from build123d import *

# Parameters (mm, degrees)
SKETCH1_R             = 22
SKETCH1_R_2           = 4
BOSS_EXTRUDE1_DEPTH   = 35
BOSS_EXTRUDE2_START   = 10
BOSS_EXTRUDE2_DEPTH   = 15
BOSS_EXTRUDE2_2_DEPTH = 15
BOSS_EXTRUDE2_3_DEPTH = 15
BOSS_EXTRUDE2_4_DEPTH = 15
SKETCH1_4_R           = 30
SKETCH1_4_R_2         = 15
SKETCH1_4_R_3         = 25
SKETCH1_4_R_4         = 10.5
BOSS_EXTRUDE3_DEPTH   = 35
BOSS_EXTRUDE5_START   = 11
BOSS_EXTRUDE5_DEPTH   = 11
SKETCH1_7_R           = 50
SKETCH1_7_R_2         = 22
BOSS_EXTRUDE6_DEPTH   = 35


with BuildPart() as part:
    # Sketch1 → Boss-Extrude1 (new body)
    with BuildSketch(Plane(origin=(0, 0, 0), x_dir=(1, 0, 0), z_dir=(0, 1, 0))):
        with Locations(Location((0, 0, 0), (0, 0, 270))):
            Circle(SKETCH1_R)
        with Locations(Location((-11.727472237, 9.352347028, 0), (0, 0, 270))):
            Circle(SKETCH1_R_2, mode=Mode.SUBTRACT)
        with Locations(Location((-14.623918683, -3.337814009, 0), (0, 0, 270))):
            Circle(SKETCH1_R_2, mode=Mode.SUBTRACT)
        with Locations(Location((-6.508256087, -13.514533019, 0), (0, 0, 270))):
            Circle(SKETCH1_R_2, mode=Mode.SUBTRACT)
        with Locations(Location((6.508256087, -13.514533019, 0), (0, 0, 270))):
            Circle(SKETCH1_R_2, mode=Mode.SUBTRACT)
        with Locations(Location((14.623918683, -3.337814009, 0), (0, 0, 270))):
            Circle(SKETCH1_R_2, mode=Mode.SUBTRACT)
        with Locations(Location((11.727472237, 9.352347028, 0), (0, 0, 270))):
            Circle(SKETCH1_R_2, mode=Mode.SUBTRACT)
        with Locations(Location((0, 15, 0), (0, 0, 270))):
            Circle(SKETCH1_R_2, mode=Mode.SUBTRACT)
    extrude(amount=BOSS_EXTRUDE1_DEPTH)



with BuildPart() as body_2:
    # Sketch1_3 → Boss-Extrude2 (new body)
    with BuildSketch(Plane(origin=(0, 0, 0), x_dir=(1, 0, 0), z_dir=(0, 1, 0)).offset(BOSS_EXTRUDE2_START)):
        with BuildLine():
            Line((-29.090909091, 49.166608302), (-135.454545455, 29.499964981))
            ThreePointArc((-135.454545455, 29.499964981), (-118.841537744, 27.847598103), (-105.684210842, 17.57106706))
            ThreePointArc((-105.684210842, 17.57106706), (-106.272845666, 22.359321946), (-102.540670225, 25.416239066))
            Line((-102.540670225, 25.416239066), (-68.238836594, 31.758650348))
            ThreePointArc((-68.238836594, 31.758650348), (-64.040683205, 30.607898174), (-62.335471097, 26.602779686))
            ThreePointArc((-62.335471097, 26.602779686), (-48.07934713, 41.370886681), (-29.090909091, 49.166608302))
        make_face()
    extrude(amount=BOSS_EXTRUDE2_DEPTH)



with BuildPart() as body_3:
    # Sketch1_3 → Boss-Extrude2 2 (new body)
    with BuildSketch(Plane(origin=(0, 0, 0), x_dir=(1, 0, 0), z_dir=(0, 1, 0)).offset(BOSS_EXTRUDE2_START)):
        with BuildLine():
            Line((65.058027183, 118.797588822), (-29.090909091, 49.166608302))
            ThreePointArc((-29.090909091, 49.166608302), (-14.295406408, 49.673510163), (0, 45.82575695))
            ThreePointArc((0, 45.82575695), (-2.026867504, 49.845767293), (0, 53.865777636))
            Line((0, 53.865777636), (50.073723573, 90.899467114))
            ThreePointArc((50.073723573, 90.899467114), (53.176128361, 91.877785359), (56.223814659, 90.740406669))
            ThreePointArc((56.223814659, 90.740406669), (56.077798236, 106.205763396), (65.058027183, 118.797588822))
        make_face()
    extrude(amount=BOSS_EXTRUDE2_2_DEPTH)


with BuildPart() as body_4:
    # Sketch1_3 → Boss-Extrude2 3 (new body)
    with BuildSketch(Plane(origin=(0, 0, 0), x_dir=(1, 0, 0), z_dir=(0, 1, 0)).offset(BOSS_EXTRUDE2_START)):
        with BuildLine():
            ThreePointArc((-105.684210842, -17.57106706), (-118.841537744, -27.847598103), (-135.454545455, -29.499964981))
            Line((-135.454545455, -29.499964981), (-29.090909091, -49.166608302))
            ThreePointArc((-29.090909091, -49.166608302), (-48.07934713, -41.370886681), (-62.335471097, -26.602779686))
            ThreePointArc((-62.335471097, -26.602779686), (-64.040683205, -30.607898174), (-68.238836594, -31.758650348))
            Line((-68.238836594, -31.758650348), (-102.540670225, -25.416239066))
            ThreePointArc((-102.540670225, -25.416239066), (-106.272845666, -22.359321946), (-105.684210842, -17.57106706))
        make_face()
    extrude(amount=BOSS_EXTRUDE2_3_DEPTH)


with BuildPart() as body_5:
    # Sketch1_3 → Boss-Extrude2 4 (new body)
    with BuildSketch(Plane(origin=(0, 0, 0), x_dir=(1, 0, 0), z_dir=(0, 1, 0)).offset(BOSS_EXTRUDE2_START)):
        with BuildLine():
            ThreePointArc((33.280664522, 3.734547986), (31.165717268, 3.098740137), (29.768218703, 4.808784369))
            ThreePointArc((29.768218703, 4.808784369), (28.343242321, -12.76443974), (20.907291105, -28.750539725))
            Line((20.907291105, -28.750539725), (100.377335216, 84.322267243))
            ThreePointArc((100.377335216, 84.322267243), (88.928428781, 75.375558771), (74.437778368, 74.306867224))
            ThreePointArc((74.437778368, 74.306867224), (78.004991776, 71.229681071), (77.43132522, 66.553679275))
            Line((77.43132522, 66.553679275), (33.280664522, 3.734547986))
        make_face()
    extrude(amount=BOSS_EXTRUDE2_4_DEPTH)


with BuildPart() as body_2_1:
    add(body_2.part)

    add(body_3.part)  # Boss-Extrude3 merges body 3

    add(body_4.part)  # Boss-Extrude3 merges body 4

    add(body_5.part)  # Boss-Extrude3 merges body 5
    # Sketch1_4 → Boss-Extrude3 (add)
    # profile 1 of 2: a face of its own
    with BuildSketch(Plane(origin=(0, 0, 0), x_dir=(1, 0, 0), z_dir=(0, 1, 0))):
        with Locations(Location((-130, 0, 0), (0, 0, 270))):
            Circle(SKETCH1_4_R)
        with Locations(Location((-130, 0, 0), (0, 0, 270))):
            Circle(SKETCH1_4_R_2, mode=Mode.SUBTRACT)
    # profile 2 of 2: a face of its own
    with BuildSketch(Plane(origin=(0, 0, 0), x_dir=(1, 0, 0), z_dir=(0, 1, 0))):
        with Locations(Location((79.923689663, 98.697537105, 0), (0, 0, 270))):
            Circle(SKETCH1_4_R_3)
        with Locations(Location((79.923689663, 98.697537105, 0), (0, 0, 270))):
            Circle(SKETCH1_4_R_4, mode=Mode.SUBTRACT)
    extrude(amount=BOSS_EXTRUDE3_DEPTH)

    # Sketch1_6 → Boss-Extrude5 (add)
    with BuildSketch(Plane(origin=(0, 0, 0), x_dir=(1, 0, 0), z_dir=(0, 1, 0)).offset(BOSS_EXTRUDE5_START)):
        with BuildLine():
            ThreePointArc((-102.540670225, 25.416239066), (-106.272845666, 22.359321946), (-105.684210842, 17.57106706))
            ThreePointArc((-105.684210842, 17.57106706), (-101.456404617, 9.233805425), (-100, 0))
            ThreePointArc((-100, 0), (-101.456404617, -9.233805425), (-105.684210842, -17.57106706))
            ThreePointArc((-105.684210842, -17.57106706), (-106.272845666, -22.359321946), (-102.540670225, -25.416239066))
            Line((-102.540670225, -25.416239066), (-68.238836594, -31.758650348))
            ThreePointArc((-68.238836594, -31.758650348), (-64.040683205, -30.607898174), (-62.335471097, -26.602779686))
            ThreePointArc((-62.335471097, -26.602779686), (-70, 0), (-62.335471097, 26.602779686))
            ThreePointArc((-62.335471097, 26.602779686), (-64.040683205, 30.607898174), (-68.238836594, 31.758650348))
            Line((-68.238836594, 31.758650348), (-102.540670225, 25.416239066))
        make_face()
        with BuildLine():
            ThreePointArc((0, 53.865777636), (-2.026867504, 49.845767293), (0, 45.82575695))
            ThreePointArc((0, 45.82575695), (20.466023961, 29.368365716), (29.768218703, 4.808784369))
            ThreePointArc((29.768218703, 4.808784369), (31.165717268, 3.098740137), (33.280664522, 3.734547986))
            Line((33.280664522, 3.734547986), (77.43132522, 66.553679275))
            ThreePointArc((77.43132522, 66.553679275), (78.004991776, 71.229681071), (74.437778368, 74.306867224))
            ThreePointArc((74.437778368, 74.306867224), (63.176515718, 80.135959455), (56.223814659, 90.740406669))
            ThreePointArc((56.223814659, 90.740406669), (53.176128361, 91.877785359), (50.073723573, 90.899467114))
            Line((50.073723573, 90.899467114), (0, 53.865777636))
        make_face()
    extrude(amount=BOSS_EXTRUDE5_DEPTH)


with BuildPart() as part_1:
    add(part.part)

    add(body_2_1.part)  # Boss-Extrude6 merges body 2
    # Sketch1_7 → Boss-Extrude6 (add)
    with BuildSketch(Plane(origin=(0, 0, 0), x_dir=(1, 0, 0), z_dir=(0, 1, 0))):
        with Locations(Location((-20, 0, 0), (0, 0, 270))):
            Circle(SKETCH1_7_R)
        Circle(SKETCH1_7_R_2, mode=Mode.SUBTRACT)
        with BuildLine():
            ThreePointArc((0.714285714, 34.218684477), (-34.403072902, 37.316906235), (-58.3325939, 11.428571429))
            ThreePointArc((-58.3325939, 11.428571429), (-57.549938291, 7.011928477), (-53.541019662, 5))
            Line((-53.541019662, 5), (-28.284271247, 5))
            ThreePointArc((-28.284271247, 5), (-25.397519902, 5.917517095), (-23.57022604, 8.333333333))
            ThreePointArc((-23.57022604, 8.333333333), (-15.064900332, 19.951159815), (-1.5625, 24.951124098))
            ThreePointArc((-1.5625, 24.951124098), (2.980616225, 28.748457023), (0.714285714, 34.218684477))
        make_face(mode=Mode.SUBTRACT)
        with BuildLine():
            ThreePointArc((-58.3325939, -11.428571429), (-34.403072902, -37.316906235), (0.714285714, -34.218684477))
            ThreePointArc((0.714285714, -34.218684477), (2.980616225, -28.748457023), (-1.5625, -24.951124098))
            ThreePointArc((-1.5625, -24.951124098), (-15.064900332, -19.951159815), (-23.57022604, -8.333333333))
            ThreePointArc((-23.57022604, -8.333333333), (-25.397519902, -5.917517095), (-28.284271247, -5))
            Line((-28.284271247, -5), (-53.541019662, -5))
            ThreePointArc((-53.541019662, -5), (-57.549938291, -7.011928477), (-58.3325939, -11.428571429))
        make_face(mode=Mode.SUBTRACT)
    extrude(amount=BOSS_EXTRUDE6_DEPTH)


solid = part_1.part
Design review of the part built by this model. Coordinates are the model's own, in mm. A direction names the side the tool comes from. Round coordinates to 2 decimals unless told otherwise and drop trailing zeros. Write each loop counter-clockwise with the first axis right and the second up, starting at its lowest first coordinate (ties: lowest second). Pieces come first, ordered by that corner, then holes.
Item 1: Consider section C-C on x = -130. Give the boundary of the cut face in (y, z), and give its area (3 significant figures).
Item 2: Draft analysis for pull direction Z (two halves, no side actions). For faces 1 (the flat face through (18, 10, -77)), 2 (the cylindrical face through (-34.88, 17.26, 37.13)), state which applies: released by +Z, released by -Z, zero draft, split by the parting line, or undercut.
Item 3: Consider section B-B on y = 3. Count the separate pieces of the cut face and the enclosed holes in it, and give its area (3 significant figures).
Item 4: Wall thickness on L1, parallel to X at y = 13, z = 0; L2, parallel to Z at x = 12, y = 21.5; L3, parallel to X at y = 19, z = -9: over which ranges is each line inside the solid? List them lowest first.
Item 5: For pin 1 Ø2 at (x, z) = (-112, 25.5) entering from -Y; pin 2 Ø22 at (x, z) = (20, -67) entering from +Y; pin 3 Ø7.5 at (x, y) = (-35, 24) entering from -Z; pin 4 Ø10.5 at (x, z) = (14.62, 3.34) entering from +Y, all flat-tipped, find the tip position at first contact; note any pin that passes through.
Item 6: Consider section A-A on z = -104.5. Give the boundary of the cut face in (x, y).
Item 7: For faces 3 (the cylindrical face through (-63.993, 10.493, 30.566)), 4 (the cylindrical face through (-63.993, 23.479, 30.566)), 5 (the cylindrical face through (-57.589, 17.255, -7.064)), list the 3-axis set-ups (+Z, -Z, +X, -X, +Y, -Y) from which the entire face can be reached by the end or side of a thin tool; tool diameter is ignored.
Check values:
1. outline: (0, -30) - (10, -30) - (10, -30.51) - (25, -30.51) - (25, -30) - (35, -30) - (35, -15) - (0, -15) - close; (0, 15) - (35, 15) - (35, 30) - (25, 30) - (25, 30.51) - (10, 30.51) - (10, 30) - (0, 30) - close
1. area: 1,070 mm2
2. face 1: zero draft
2. face 2: undercut
3. separate pieces: 3
3. enclosed holes: 11
3. area: 8,510 mm2
4. L1: x = -160 to -145, -115 to -16.83, -12.42 to 12.42, 16.83 to 41.11
4. L2: z = -79.56 to -13.34, -5.36 to 0.32, 6.36 to 38.42
4. L3: x = -158.62 to -142, -118 to -58.44, -23.32 to -15.71, -7.74 to 7.74, 15.71 to 47.44
5. pin 1: stops at y = 10
5. pin 2: stops at y = 25
5. pin 3: stops at z = -48.77
5. pin 4: stops at y = 35
6. outline: (45.73, 10) - (55.61, 10) - (55.61, 0) - (71.17, 0) - (71.17, 35) - (55.61, 35) - (55.61, 25) - (45.73, 25) - close; (88.67, 0) - (104.24, 0) - (104.24, 35) - (88.67, 35) - close
7. face 3: -Y
7. face 4: +Y
7. face 5: +Y, -Y
